Read the model definition and answer for the solid it produces. Units are mm, in the model's axes. Face numbers are marked on the shaded views. A direction names the side the tool comes from. Coordinates: 2 decimals unless noted, no trailing zeros. Loops run counter-clockwise (first coordinate to the right, second up) from the corner with the lowest first, then second, coordinate; pieces in that order, holes last.
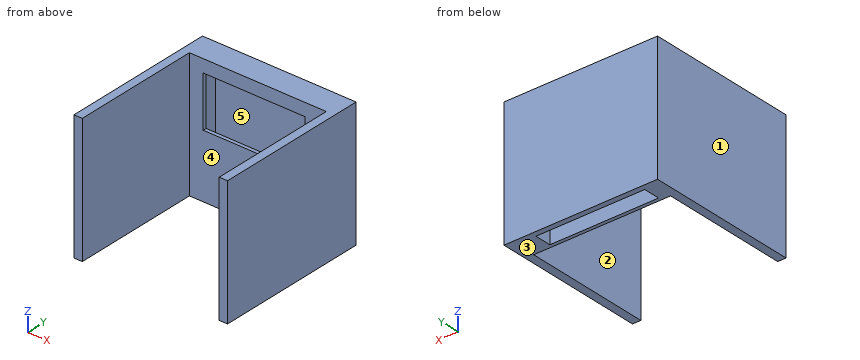
from build123d import *

# Parameters (mm, degrees)
SKETCH1_W           = 120
SKETCH1_H           = 100
BOSS_EXTRUDE1_DEPTH = 120
SKETCH2_W           = 107
SKETCH2_H           = 120
CUT_EXTRUDE1_DEPTH  = 100
SKETCH4_W           = 85
SKETCH4_H           = 13
CUT_EXTRUDE2_DEPTH  = 95
CUT_EXTRUDE3_START  = -50
SKETCH5_W           = 79.569660058
SKETCH5_H           = 2.731854476
CUT_EXTRUDE3_DEPTH  = 40


with BuildPart() as part:
    # Sketch1 → Boss-Extrude1 (new body)
    with BuildSketch(Plane(origin=(0, 0, 0), x_dir=(1, 0, 0), z_dir=(0, 1, 0))):
        Rectangle(SKETCH1_W, SKETCH1_H)
    extrude(amount=BOSS_EXTRUDE1_DEPTH)

    # Sketch2 → Cut-Extrude1 (cut)
    with BuildSketch(Plane.XZ):
        Rectangle(SKETCH2_W, SKETCH2_H)
    extrude(amount=-CUT_EXTRUDE1_DEPTH, mode=Mode.SUBTRACT)

    # Sketch4 → Cut-Extrude2 (cut)
    with BuildSketch(Plane(origin=(0, 0, -50), x_dir=(-1, 0, 0), z_dir=(0, 0, -1))):
        with Locations((3.915635034, 109.231854476)):
            Rectangle(SKETCH4_W, SKETCH4_H)
    extrude(amount=-CUT_EXTRUDE2_DEPTH, mode=Mode.SUBTRACT)

    # Sketch5 → Cut-Extrude3 (cut)
    with BuildSketch(Plane(origin=(0, 0, -50), x_dir=(-1, 0, 0), z_dir=(0, 0, -1)).offset(CUT_EXTRUDE3_START)):
        with Locations((2.947024447, 101.365927238)):
            Rectangle(SKETCH5_W, SKETCH5_H)
    extrude(amount=-CUT_EXTRUDE3_DEPTH, mode=Mode.SUBTRACT)


solid = part.part
Q1. A cutting plane is placed at C-C (z = -8.5). Give the vertices of the cut face in (x, y).
Findings below:
outline: (-60, 0) - (-53.5, 0) - (-53.5, 100) - (53.5, 100) - (53.5, 0) - (60, 0) - (60, 120) - (-60, 120) - close; hole (-46.42, 102.73) - (38.58, 102.73) - (38.58, 115.73) - (-46.42, 115.73) - close
Q2. Flat-ended cylindrical pins translate along their axes: pin 1 Ø6.5 at (x, y) = (10, 110.5) entering from -Z; pin 2 Ø1.5 at (x, y) = (28, 99.5) entering from +Z; pin 3 Ø4 at (x, z) = (13.5, -15.5) entering from -Y. Find the tip coordinate at first contact, or state that the pin passes through.
Findings below:
pin 1: stops at z = 45
pin 2: stops at z = 50
pin 3: stops at y = 100
Q3. A cutting plane is placed at A-A (y = 33). Give the vertices of the cut face in (x, z).
Findings below:
outline: (-60, -50) - (-53.5, -50) - (-53.5, 50) - (-60, 50) - close; (53.5, -50) - (60, -50) - (60, 50) - (53.5, 50) - close
Q4. A cutting plane is placed at B-B (x = 9). Give the vertices of the cut face in (y, z).
Findings below:
outline: (100, -50) - (102.73, -50) - (102.73, 0) - (100, 0) - close; (100, 40) - (102.73, 40) - (102.73, 45) - (115.73, 45) - (115.73, -50) - (120, -50) - (120, 50) - (100, 50) - close
Q5. A cutting plane is placed at D-D (z = 13). Give the vertices of the cut face in (x, y).
Findings below:
outline: (-60, 0) - (-53.5, 0) - (-53.5, 100) - (-42.73, 100) - (-42.73, 102.73) - (-46.42, 102.73) - (-46.42, 115.73) - (38.58, 115.73) - (38.58, 102.73) - (36.84, 102.73) - (36.84, 100) - (53.5, 100) - (53.5, 0) - (60, 0) - (60, 120) - (-60, 120) - close
Q6. Determine the mould class of the marked faces 3, 4 and 5 for opening direction Y: +Y half, -Y half, draft (parallel to the pull), parting line (faces both ways), or undercut.
Findings below:
face 3: draft
face 4: -Y half
face 5: undercut
Q7. Straight lines are drawn through the part: probe 1 along X at (y, z) = (110.5, 16.5); probe 2 along X at (y, z) = (58, 39); probe 3 along Y at (x, z) = (-26, -26.5). For each, find the intervals that lie inside material, in ascending order.
Findings below:
probe 1: x = -60 to -46.42, 38.58 to 60
probe 2: x = -60 to -53.5, 53.5 to 60
probe 3: y = 100 to 102.73, 115.73 to 120
Q8. Which of the six approach directions +Z, -Z, +X, -X, +Y, -Y give full straight-line access (tool end or side, diameter ignored) to the marked faces 1 and 2?
Findings below:
face 1: +Z, -Z, -X, +Y, -Y
face 2: +Z, -Z, -Y
